Geometry check sheet. Reference: the model listing, model coordinates, mm. A direction names the side the tool comes from. Give positions to 0.01 mm unless a question says otherwise; leave off trailing zeros. Write each loop counter-clockwise with the first axis right and the second up, starting at its lowest first coordinate (ties: lowest second). Pieces come first, ordered by that corner, then holes. Notation, with made-up numbers: (6.25, 45.25) -> (60.25, 45.25) arc R20 cw to (60.25, 61.25) -> close; hole circle Ø11 at (-33, -15.5). An arc over 180 degrees is marked (long way). One line per item, written item: value.
Autodesk Inventor part; units mm, degrees
ref_plane "YZ Plane" through (0, 0, 0) normal (1, 0, 0) x (0, 1, 0)
ref_plane "XZ Plane" through (0, 0, 0) normal (0, 1, 0) x (-1, 0, 0)
ref_plane "XY Plane" through (0, 0, 0) normal (0, 0, 1) x (1, 0, 0)
sketch "Sketch1" plane through (0, 0, 0) normal (0, 1, 0) x (-1, 0, 0)
  line L0 (-30, 10) -> (30, 10)
  line L1 (30, 10) -> (30, -10)
  line L2 (30, -10) -> (-30, -10)
  line L3 (-30, -10) -> (-30, 10)
  point P0 (0, 0)
  point P1 (30, 0)
  point P2 (0, 10)
  dimension "d0" = 60
  dimension "d1" = 20
extrude "Extrusion1" add sketch "Sketch1" along normal blind 10
sketch "Sketch2" plane through (0, 10, 0) normal (0, 1, 0) x (1, 0, 0)
  line L0 (27.75, -7.75) -> (22.25, -7.75)
  line L1 (22.25, -7.75) -> (22.25, -2.25)
  line L2 (22.25, -2.25) -> (27.75, -2.25)
  line L3 (27.75, -2.25) -> (27.75, -7.75)
  line L4 (30, -10) -> (30, 10)
  line L5 (-30, -10) -> (30, -10)
  line L6 (12.2, -7.8) -> (17.8, -7.8)
  line L7 (17.8, -7.8) -> (17.8, -2.2)
  line L8 (17.8, -2.2) -> (12.2, -2.2)
  line L9 (12.2, -2.2) -> (12.2, -7.8)
  line L10 (2.15, -7.85) -> (7.85, -7.85)
  line L11 (7.85, -7.85) -> (7.85, -2.15)
  line L12 (7.85, -2.15) -> (2.15, -2.15)
  line L13 (2.15, -2.15) -> (2.15, -7.85)
  line L14 (-7.9, -7.9) -> (-2.1, -7.9)
  line L15 (-2.1, -7.9) -> (-2.1, -2.1)
  line L16 (-2.1, -2.1) -> (-7.9, -2.1)
  line L17 (-7.9, -2.1) -> (-7.9, -7.9)
  line L18 (-17.95, -7.95) -> (-12.05, -7.95)
  line L19 (-12.05, -7.95) -> (-12.05, -2.05)
  line L20 (-12.05, -2.05) -> (-17.95, -2.05)
  line L21 (-17.95, -2.05) -> (-17.95, -7.95)
  line L22 (-28, -8) -> (-22, -8)
  line L23 (-22, -8) -> (-22, -2)
  line L24 (-22, -2) -> (-28, -2)
  line L25 (-28, -2) -> (-28, -8)
  point P0 (0, 0)
  point P1 (-12.05, -5)
  point P2 (-7.9, -5)
  point P3 (-2.1, -5)
  point P4 (2.15, -5)
  point P5 (7.85, -5)
  point P6 (12.2, -5)
  point P7 (17.8, -5)
  point P8 (22.25, -5)
  point P9 (15, -7.8)
  point P10 (25, -7.75)
  point P11 (5, -7.85)
  point P12 (-5, -7.9)
  point P13 (-15, -7.95)
  point P14 (-25, -8)
  point P15 (-22, -5)
  point P16 (-17.95, -5)
  dimension "d9" = 5.5
  dimension "d10" = 5.6
  dimension "d11" = 5.7
  dimension "d12" = 5.8
  dimension "d13" = 5.9
  dimension "d14" = 10
  dimension "d15" = 10
  dimension "d16" = 10
  dimension "d17" = 10
  dimension "d18" = 5
  dimension "d19" = 6
  dimension "d20" = 10
  dimension "d65" = 5
extrude "Extrusion2" cut sketch "Sketch2" against normal blind 1.8
sketch "Sketch3" plane through (-30, 0, 10) normal (0, 0, 1) x (1, 0, 0)
  line L0 (2, 6.15) -> (8, 6.15)
  line L1 (8, 6.15) -> (8, 3.85)
  line L2 (8, 3.85) -> (2, 3.85)
  line L3 (2, 3.85) -> (2, 6.15)
  line L4 (12, 6.1) -> (18, 6.1)
  line L5 (18, 6.1) -> (18, 3.9)
  line L6 (18, 3.9) -> (12, 3.9)
  line L7 (12, 3.9) -> (12, 6.1)
  line L8 (22, 6.05) -> (28, 6.05)
  line L9 (28, 6.05) -> (28, 3.95)
  line L10 (28, 3.95) -> (22, 3.95)
  line L11 (22, 3.95) -> (22, 6.05)
  line L12 (32, 6) -> (38, 6)
  line L13 (38, 6) -> (38, 4)
  line L14 (38, 4) -> (32, 4)
  line L15 (32, 4) -> (32, 6)
  line L16 (42, 5.95) -> (48, 5.95)
  line L17 (48, 5.95) -> (48, 4.05)
  line L18 (48, 4.05) -> (42, 4.05)
  line L19 (42, 4.05) -> (42, 5.95)
  line L20 (52, 5.9) -> (58, 5.9)
  line L21 (58, 5.9) -> (58, 4.1)
  line L22 (58, 4.1) -> (52, 4.1)
  line L23 (52, 4.1) -> (52, 5.9)
  line L24 (60, 0) -> (60, 10)
  point P0 (30, 0)
  point P1 (55, 5.9)
  point P2 (45, 5.95)
  point P3 (35, 6)
  point P4 (25, 6.05)
  point P5 (15, 6.1)
  point P6 (5, 6.15)
  point P7 (8, 5)
  point P8 (12, 5)
  point P9 (18, 5)
  point P10 (22, 5)
  point P11 (28, 5)
  point P12 (32, 5)
  point P13 (38, 5)
  point P14 (42, 5)
  point P15 (48, 5)
  point P16 (52, 5)
  point P17 (58, 5)
  point P18 (60, 5)
  dimension "d23" = 6
  dimension "d24" = 1.8
  dimension "d25" = 5
  dimension "d26" = 10
  dimension "d27" = 10
  dimension "d28" = 10
  dimension "d29" = 10
  dimension "d30" = 10
  dimension "d31" = 1.9
  dimension "d32" = 2
  dimension "d33" = 2.1
  dimension "d34" = 2.2
  dimension "d35" = 2.3
extrude "Extrusion3" cut sketch "Sketch3" against normal blind 6
sketch "Sketch4" plane through (0, 0, 0) normal (0, -1, 0) x (1, 0, 0)
  line L0 (27.75, 2.25) -> (22.25, 2.25)
  line L1 (22.25, 2.25) -> (22.25, 7.75)
  line L2 (22.25, 7.75) -> (27.75, 7.75)
  line L3 (27.75, 7.75) -> (27.75, 2.25)
  line L4 (12.2, 2.2) -> (17.8, 2.2)
  line L5 (17.8, 2.2) -> (17.8, 7.8)
  line L6 (17.8, 7.8) -> (12.2, 7.8)
  line L7 (12.2, 7.8) -> (12.2, 2.2)
  line L8 (2.15, 2.15) -> (7.85, 2.15)
  line L9 (7.85, 2.15) -> (7.85, 7.85)
  line L10 (7.85, 7.85) -> (2.15, 7.85)
  line L11 (2.15, 7.85) -> (2.15, 2.15)
  line L12 (-7.9, 2.1) -> (-2.1, 2.1)
  line L13 (-2.1, 2.1) -> (-2.1, 7.9)
  line L14 (-2.1, 7.9) -> (-7.9, 7.9)
  line L15 (-7.9, 7.9) -> (-7.9, 2.1)
  line L16 (-17.95, 2.05) -> (-12.05, 2.05)
  line L17 (-12.05, 2.05) -> (-12.05, 7.95)
  line L18 (-12.05, 7.95) -> (-17.95, 7.95)
  line L19 (-17.95, 7.95) -> (-17.95, 2.05)
  line L20 (-28, 2) -> (-22, 2)
  line L21 (-22, 2) -> (-22, 8)
  line L22 (-22, 8) -> (-28, 8)
  line L23 (-28, 8) -> (-28, 2)
  line L24 (30, 10) -> (-30, 10)
  line L25 (30, -10) -> (30, 10)
  point P0 (0, 0)
  point P1 (-12.05, 5)
  point P2 (-7.9, 5)
  point P3 (-2.1, 5)
  point P4 (2.15, 5)
  point P5 (7.85, 5)
  point P6 (12.2, 5)
  point P7 (17.8, 5)
  point P8 (22.25, 5)
  point P9 (15, 2.2)
  point P10 (25, 2.25)
  point P11 (5, 2.15)
  point P12 (-5, 2.1)
  point P13 (-15, 2.05)
  point P14 (-25, 2)
  point P15 (-22, 5)
  point P16 (-17.95, 5)
  dimension "d38" = 5.5
  dimension "d39" = 5.6
  dimension "d40" = 5.7
  dimension "d41" = 5.8
  dimension "d42" = 5.9
  dimension "d43" = 10
  dimension "d44" = 10
  dimension "d45" = 10
  dimension "d46" = 10
  dimension "d47" = 6
  dimension "d48" = 10
  dimension "d51" = 5
  dimension "d53" = 5
extrude "Extrusion4" cut sketch "Sketch4" against normal blind 1.8
hole "Hole1" at (25, 10, -5) direction (0, -1, 0) diameter 3 end through all counterbore diameter 5.5 counterbore depth 3
hole "Hole2" at (15, 10, -5) direction (0, -1, 0) diameter 3.1 end through all counterbore diameter 5.6 counterbore depth 3.1
hole "Hole3" at (5, 10, -5) direction (0, -1, 0) diameter 3.2 end through all counterbore diameter 5.7 counterbore depth 3.2
hole "Hole4" at (-5, 10, -5) direction (0, -1, 0) diameter 3.3 end through all counterbore diameter 5.8 counterbore depth 3.3
hole "Hole5" at (-15, 10, -5) direction (0, -1, 0) diameter 3.4 end through all counterbore diameter 5.9 counterbore depth 3.4
hole "Hole6" at (-25, 10, -5) direction (0, -1, 0) diameter 3.5 end through all counterbore diameter 6 counterbore depth 3.5
equation "\"d9\" = nut_A"
equation "\"d21\" = nut_B"
equation "\"d24\" = nut_B"
equation "\"d38\" = d49"
equation "\"d54\" = nut_B"
equation "\"d58\" = screw_m3_A"
equation "\"d60\" = screw_m3_C"
equation "\"d61\" = screw_m3_D"
properties part number "TOLERANCE_TEST"
1) Mould release check, pull along Z, two halves, no side actions. Record for faces 5 (the flat face through (-7.9, 9, 5)), 6 (the flat face through (25, 4.1, 7)), 7 (the flat face through (25, 5, 4)): released by +Z, released by -Z, zero draft, split by the parting line, or undercut.
Verdict:
face 5: undercut
face 6: zero draft
face 7: released by +Z
2) Sectioned sample at D-D on x = -5. Record the cut outline in (y, z), plus the area to 3 significant figures.
Verdict:
outline: (0, -10) -> (10, -10) -> (10, -7.9) -> (6.7, -7.9) -> (6.7, -6.65) -> (0, -6.65) -> close; (0, -3.35) -> (6.7, -3.35) -> (6.7, -2.1) -> (10, -2.1) -> (10, 2.1) -> (8.2, 2.1) -> (8.2, 7.9) -> (10, 7.9) -> (10, 10) -> (6.05, 10) -> (6.05, 4) -> (3.95, 4) -> (3.95, 10) -> (0, 10) -> (0, 7.9) -> (1.8, 7.9) -> (1.8, 2.1) -> (0, 2.1) -> close
area: 125 mm^2
3) Scan lines: probe 1 along Z at (x, y) = (-17, 1.25); probe 2 along Z at (x, y) = (-25, 8.5); probe 3 along Z at (x, y) = (-15, 9.1). Record each from-to range of solid material in increasing order.
Verdict:
probe 1: -10 to 2.05, 7.95 to 10
probe 2: -10 to -8, -2 to 2, 8 to 10
probe 3: -10 to -7.95, -2.05 to 2.05, 7.95 to 10
4) Tool access check on faces 1 (the flat face through (-2.1, 1, 5)), 2 (the flat face through (-5, 6.05, 7)), 3 (the flat face through (0, 0, 0)), 4 (the flat face through (-17.95, 9, 5)). Record the directions out of +Z, -Z, +X, -X, +Y, -Y that give a thin tool (end or side, any length) a straight path to the whole face; none if there is none.
Verdict:
face 1: -Y
face 2: +Z
face 3: +Z, -Z, +X, -X, -Y
face 4: +Y
5) Sectioned sample at B-B on y = 5. Give the number of separate pieces and of enclosed holes in the cut face, plus the area to 3 significant figures.
Verdict:
separate pieces: 1
enclosed holes: 6
area: 934 mm^2
6) Sectioned sample at A-A on x = 15. Record the cut outline in (y, z).
Verdict:
outline: (0, -10) -> (10, -10) -> (10, -7.8) -> (6.9, -7.8) -> (6.9, -6.55) -> (0, -6.55) -> close; (0, -3.45) -> (6.9, -3.45) -> (6.9, -2.2) -> (10, -2.2) -> (10, 2.2) -> (8.2, 2.2) -> (8.2, 7.8) -> (10, 7.8) -> (10, 10) -> (5.95, 10) -> (5.95, 4) -> (4.05, 4) -> (4.05, 10) -> (0, 10) -> (0, 7.8) -> (1.8, 7.8) -> (1.8, 2.2) -> (0, 2.2) -> close
7) Depth check by flat-ended pin: pin 1 Ø7 at (x, z) = (25, -5) entering from -Y; pin 2 Ø1.7 at (x, z) = (3.5, 4) entering from -Y; pin 3 Ø1.7 at (x, z) = (-4.5, -4) entering from +Y. Enter the tip coordinate at first touch or a pass-through.
Verdict:
pin 1: y = 0
pin 2: y = 1.8
pin 3: y = 6.7
